Job drawing, mm, ordinate dimensions from the low corner. One solid piece. Coordinates: 2 decimals unless noted, no trailing zeros. Loops run counter-clockwise (first coordinate to the right, second up) from the corner with the lowest first, then second, coordinate; pieces in that order, holes last. Notation, with made-up numbers: (11, 59) -> (32, 59) arc R19 ccw to (32, 83) -> close; hole circle Ø5 at (-18.5, -4). An arc over 180 degrees is marked (long way). Use one line per item in the form item = value. Start each with the question number.
(1) Band-saw the part on A-A on x = 7. Give the cut face in (y, z).
(2) Band-saw the part on B-B on z = 60. Give the cut face in (x, y), then the cut area to 3 significant figures.
(3) Pin check, flat tip, straight feed: P1, Ø2.5, axis at x = 70.78, z = 18, coming from the +Y side. Stop position of the tip, or through.
(4) Drill centre lines: L1, parallel to X at y = 1.1, z = 18; L2, parallel to X at y = 1.65, z = 60. Where is each one in solid material? Low to high. Write a range as [from, to].
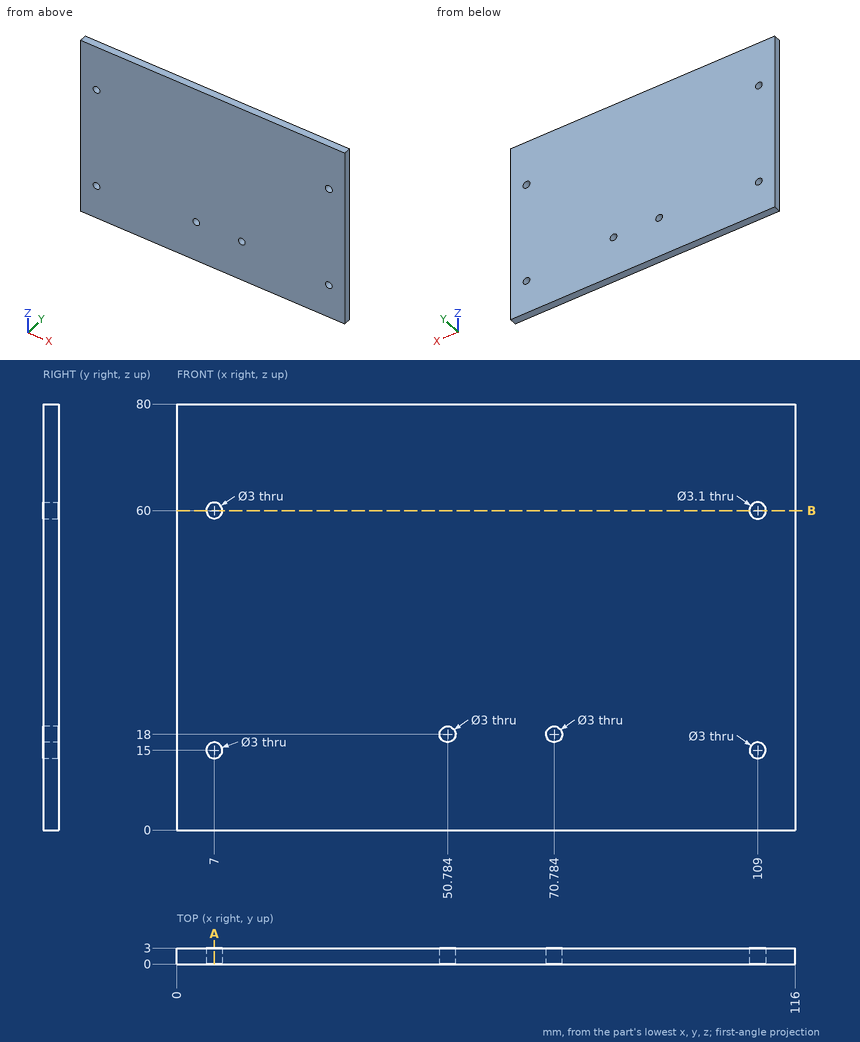
A:
q1.outline = (0, 0) -> (3, 0) -> (3, 13.5) -> (0, 13.5) -> close; (0, 16.5) -> (3, 16.5) -> (3, 58.5) -> (0, 58.5) -> close; (0, 61.5) -> (3, 61.5) -> (3, 80) -> (0, 80) -> close
q2.outline = (0, 0) -> (5.5, 0) -> (5.5, 3) -> (0, 3) -> close; (8.5, 0) -> (107.45, 0) -> (107.45, 3) -> (8.5, 3) -> close; (110.55, 0) -> (116, 0) -> (116, 3) -> (110.55, 3) -> close
q2.area = 330 mm²
q3.P1 = through
q4.L1 = [0, 49.28], [52.28, 69.28], [72.28, 116]
q4.L2 = [0, 5.5], [8.5, 107.45], [110.55, 116]
